Autodesk Inventor part; units mm, degrees
ref_plane "YZ Plane" through (0, 0, 0) normal (1, 0, 0) x (0, 1, 0)
ref_plane "XZ Plane" through (0, 0, 0) normal (0, 1, 0) x (-1, 0, 0)
ref_plane "XY Plane" through (0, 0, 0) normal (0, 0, 1) x (1, 0, 0)
sketch "Sketch1" plane through (0, 0, 0) normal (0, 1, 0) x (-1, 0, 0)
  line L0 (1.7293, -2.0233) -> (-49.0707, -2.0233)
  line L1 (-49.0707, -2.0233) -> (-49.0707, 810.7767)
  line L2 (-49.0707, 810.7767) -> (1.7293, 810.7767)
  line L3 (1.7293, 810.7767) -> (1.7293, -2.0233)
  point P0 (0, 0)
  dimension "d0" = 50.8
  dimension "d1" = 812.8
extrude "Extrusion1" add sketch "Sketch1" along normal blind 50.8
sketch "Sketch2" plane through (0, 50.8, 0) normal (0, 1, 0) x (1, 0, 0)
  line L0 (49.0707, 2.0233) -> (-1.7293, 2.0233)
  line L1 (-1.7293, 2.0233) -> (1.4457, 2.0233)
  line L2 (49.0707, 2.0233) -> (45.8957, 2.0233)
  line L3 (1.4457, 2.0233) -> (45.8957, 2.0233)
  line L4 (45.8957, 2.0233) -> (45.8957, -810.7767)
  line L5 (45.8957, -810.7767) -> (1.4457, -810.7767)
  line L6 (1.4457, -810.7767) -> (1.4457, 2.0233)
  point P0 (0, 0)
  dimension "d4" = 3.175
  dimension "d5" = 3.175
  dimension "d6" = 44.45
  dimension "d7" = 812.8
extrude "Extrusion2" cut sketch "Sketch2" against normal blind 47.625
sketch "Sketch3" plane through (49.0707, 0, 810.7767) normal (1, 0, 0) x (0, 0, -1)
  line L0 (0, 0) -> (0, 50.8)
  line L1 (0, 25.4) -> (19.05, 25.4)
  circle A0 centre (19.05, 25.4) radius 14.2875
  line L2 (19.05, 25.4) -> (76.2, 25.4)
  circle A1 centre (76.2, 25.4) radius 14.2875
  line L3 (76.2, 25.4) -> (107.95, 25.4)
  circle A2 centre (107.95, 25.4) radius 14.2875
  point P0 (810.7767, 0)
  dimension "d10" = 19.05
  dimension "d11" = 28.575
  dimension "d12" = 57.15
  dimension "d13" = 28.575
  dimension "d14" = 31.75
  dimension "d15" = 28.575
extrude "Extrusion3" cut sketch "Sketch3" against normal blind 76.2
sketch "Sketch4" plane through (49.0707, 0, 810.7767) normal (1, 0, 0) x (0, 0, -1)
  line L0 (812.8, 50.8) -> (812.8, 3.175)
  line L1 (812.8, 26.9875) -> (781.05, 26.9875)
  circle A0 centre (781.05, 26.9875) radius 14.2875
  point P0 (810.7767, 0)
  dimension "d18" = 31.75
  dimension "d19" = 28.575
extrude "Extrusion4" cut sketch "Sketch4" against normal blind 76.2
properties part number "36in Aluminum Channel"
The listing builds one solid part. Answer for the finished solid, in the listing's coordinates (mm). A direction names the side the tool comes from. Round coordinates to 2 decimals unless told otherwise and drop trailing zeros. Order: outer loops, then holes, each group sorted by start corner. A loop starts at its lowest first (then second) coordinate and runs counter-clockwise, first axis right, second up. Notation, with made-up numbers: (2.25, 65.5) -> (50.25, 65.5) arc R21 ccw to (50.25, 91.5) -> close; hole circle Ø4 at (72, -39.5). An arc over 180 degrees is marked (long way). Answer as CSV lines item,"result". Start each with the question number.
(1) The part is cut by section A-A (z = 440.5). Determine the outline of the cut face in (x, y) (3 decimals), then the cut area to 3 significant figures.
(2) A tool of negligible diameter and unlimited length cuts with its end or side. For faces 5 (the face through (23, 3.175, 399)), 6 (the face through (24, 0, 410)), from which of +Z, -Z, +X, -X, +Y, -Y can it reach the whole face along a straight path? Write none if from no direction.
(3) For a pull along X with two mould halves and no side action, classify faces 1 (the face through (45.896, 27, 399)), 2 (the face through (1.446, 27, 410)), 3 (the face through (-0.12, 19.928, 778.529)), 4 (the face through (49.071, 25, 399)) as +X half, -X half, draft (parallel to the pull), parting line (faces both ways), or undercut.
(4) Find the intervals of material crossed by probe 1 along Z at (x, y) = (0, 25); probe 2 along Z at (x, y) = (47.75, 25.4); probe 3 along X at (y, z) = (34, 132), in increasing order. Write a range as from..to.
(5) The part is cut by section B-B (x = 36). Determine the outline of the cut face in (y, z) (3 decimals), then the cut area to 3 significant figures.
(6) Flat-ended cylindrical pins translate along their axes: pin 1 Ø23 at (y, z) = (25.4, 734.58) entering from -X; pin 2 Ø2 at (x, z) = (25, 314) entering from +Y (3 decimals). Find the tip coordinate at first contact, or state that the pin passes through.
Evaluation:
1,outline,"(-1.729, 0) -> (49.071, 0) -> (49.071, 50.8) -> (45.896, 50.8) -> (45.896, 3.175) -> (1.446, 3.175) -> (1.446, 50.8) -> (-1.729, 50.8) -> close"
1,area,"464 mm²"
2,face 5,"+Z, -Z, +Y"
2,face 6,"+Z, -Z, +X, -X, -Y"
3,face 1,"undercut"
3,face 2,"undercut"
3,face 3,"draft"
3,face 4,"+X half"
4,probe 1,"-2.02..15.58, 43.88..688.54, 717.11..720.29, 748.86..777.44, 806.01..810.78"
4,probe 2,"-2.02..15.53, 43.93..688.54, 717.11..720.29, 748.86..777.44, 806.01..810.78"
4,probe 3,"-1.73..1.45, 45.9..49.07"
5,outline,"(0, -2.023) -> (3.175, -2.023) -> (3.175, 810.777) -> (0, 810.777) -> close"
5,area,"2,580 mm²"
6,pin 1,"through"
6,pin 2,"y = 3.175"
